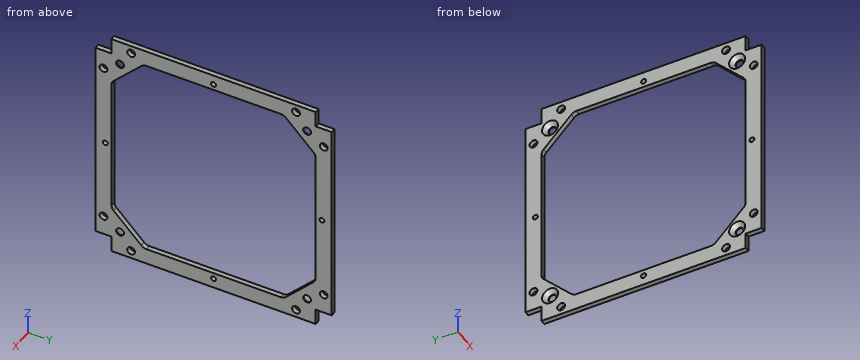
```python
from build123d import *

# Parameters (mm, degrees)
BOSS_EXTRUDE2_DEPTH                          = 2
F_3_2_3_2_DIAMETER_HOLE3_D                   = 3.2
CSK_FOR_M3_FLAT_COUNTERSUNK_HEAD_SCR_2_COUNT = 2
CSK_FOR_M3_FLAT_COUNTERSUNK_HEAD_SCR_2_PITCH = 76
CSK_FOR_M3_FLAT_COUNTERSUNK_HEAD_SCR_3_COUNT = 2
CSK_FOR_M3_FLAT_COUNTERSUNK_HEAD_SCR_3_PITCH = 107.48023074
CSK_FOR_M3_FLAT_COUNTERSUNK_HEAD_SCR_4_COUNT = 2
CSK_FOR_M3_FLAT_COUNTERSUNK_HEAD_SCR_4_PITCH = 76
M2_5X0_45_TAPPED_HOLE1_D                     = 2.05
FILLET1_R                                    = 3


with BuildPart() as part:
    # Sketch2 → Boss-Extrude2 (new body)
    with BuildSketch(Plane.ZY.offset(51.493641502)):
        Polygon((0.93465612, 3.45185693), (7.43465612, 3.45185693), (7.43465612, 86.45185693), (0.93465612, 86.45185693), (0.93465612, 92.95185693), (-82.06534388, 92.95185693), (-82.06534388, 86.45185693), (-88.56534388, 86.45185693), (-88.56534388, 3.45185693), (-82.06534388, 3.45185693), (-82.06534388, -3.04814307), (0.93465612, -3.04814307), align=None)
        Polygon((-82.06534388, 73.45185693), (-82.06534388, 16.45185693), (-69.06534388, 3.45185693), (-12.06534388, 3.45185693), (0.93465612, 16.45185693), (0.93465612, 73.45185693), (-12.06534388, 86.45185693), (-69.06534388, 86.45185693), align=None, mode=Mode.SUBTRACT)
    extrude(amount=BOSS_EXTRUDE2_DEPTH)

    # Ø3.2 (3.2) Diameter Hole3 (through all)
    with Locations(Plane.ZY.offset(53.493641502)):
        with Locations((-74.06534388, 0.20185693), (-85.31534388, 11.45185693), (-85.31534388, 78.45185693), (-74.06534388, 89.70185693), (-7.06534388, 89.70185693), (4.18465612, 78.45185693), (4.18465612, 11.45185693), (-7.06534388, 0.20185693)):
            Hole(F_3_2_3_2_DIAMETER_HOLE3_D / 2)

    # Sketch24 → CSK for M3 Flat Countersunk Head Screw5 (revolve, cut)
    with BuildSketch(Plane(origin=(-53.493641502, 6.95185693, -78.56534388), x_dir=(0, 0, 1), z_dir=(0, 1, 0))):
        Polygon((0, 0), (0, 2), (1.6, 2), (1.6, 1.65), (3.25, 0), align=None)
    csk_for_m3_flat_countersunk_head_screw5 = revolve(axis=Axis((-59.843641502, 6.95185693, -78.56534388), (1, 0, 0)), mode=Mode.SUBTRACT)

    # CSK for M3 Flat Countersunk Head Scr 2: CSK for M3 Flat Countersunk Head Screw5 ×2
    with Locations(*[(0, i * CSK_FOR_M3_FLAT_COUNTERSUNK_HEAD_SCR_2_PITCH, 0) for i in range(1, CSK_FOR_M3_FLAT_COUNTERSUNK_HEAD_SCR_2_COUNT)]):
        add(csk_for_m3_flat_countersunk_head_screw5, mode=Mode.SUBTRACT)

    # CSK for M3 Flat Countersunk Head Scr 3: CSK for M3 Flat Countersunk Head Screw5 ×2
    with Locations(*[Vector(0, 0.7071067811865478, 0.7071067811865472) * (i * CSK_FOR_M3_FLAT_COUNTERSUNK_HEAD_SCR_3_PITCH) for i in range(1, CSK_FOR_M3_FLAT_COUNTERSUNK_HEAD_SCR_3_COUNT)]):
        add(csk_for_m3_flat_countersunk_head_screw5, mode=Mode.SUBTRACT)

    # CSK for M3 Flat Countersunk Head Scr 4: CSK for M3 Flat Countersunk Head Screw5 ×2
    with Locations(*[(0, 0, i * CSK_FOR_M3_FLAT_COUNTERSUNK_HEAD_SCR_4_PITCH) for i in range(1, CSK_FOR_M3_FLAT_COUNTERSUNK_HEAD_SCR_4_COUNT)]):
        add(csk_for_m3_flat_countersunk_head_screw5, mode=Mode.SUBTRACT)

    # M2.5x0.45 Tapped Hole1 (through all)
    with Locations(Plane(origin=(-53.493641502, 88.95185693, -40.56534388), x_dir=(0, 0, -1), z_dir=(-1, 0, 0))):
        with Locations((0, 0), (44, 44), (0, 88), (-44, 44)):
            Hole(M2_5X0_45_TAPPED_HOLE1_D / 2)

    # Fillet1
    fillet1_edges = [part.edges().sort_by_distance(p)[0] for p in [
        (-52.493641502, 86.45185693, -69.06534388),
        (-52.493641502, 73.45185693, -82.06534388),
        (-52.493641502, 16.45185693, -82.06534388),
        (-52.493641502, 3.45185693, -69.06534388),
        (-52.493641502, 3.45185693, -12.06534388),
        (-52.493641502, 16.45185693, 0.93465612),
        (-52.493641502, 73.45185693, 0.93465612),
        (-52.493641502, 86.45185693, -12.06534388),
    ]]
    fillet(fillet1_edges, radius=FILLET1_R)


solid = part.part
```
CAD build for the part. Positions are in the model's coordinates, mm. Coordinates: 2 decimals unless noted, no trailing zeros. Write each loop counter-clockwise with the first axis right and the second up, starting at its lowest first coordinate (ties: lowest second). Pieces come first, ordered by that corner, then holes. Notation, with made-up numbers: (20.5, -14) -> (63.5, -14) arc R29 ccw to (63.5, 7) -> close; hole circle Ø5 at (40, -34.5). An arc over 180 degrees is marked (long way). Use CSV: the item, a comma, the result in double quotes. Start each with the question number.
Item 1: Band-saw the part on A-A, the plane y = 35.5. Write the cut outline in (x, z).
Item 2: Drop flat-ended pins along their axis: P1, Ø4, axis at y = 0.2, z = -74.07, coming from the +X side; P2, Ø0.6, axis at x = -52, z = 2.5, coming from the -Y side. Give the stop position or say it passes through.
Item 3: Band-saw the part on B-B, the plane z = -55. Write the cut outline in (x, y), plus the area to 3 significant figures.
Item 4: Band-saw the part on C-C, the plane x = -53.1. Give the number of separate pieces and of enclosed holes in the cut face, plus the area to 3 significant figures.
Item 5: Wall check: probe 1 along Y at (x, z) = (-51.8, -43); probe 2 along Z at (x, y) = (-52.45, 27); probe 3 along Y at (x, z) = (-52.7, -79.5). Give the ranges that are in metal, low to high.
Response values:
1,outline,"(-53.49, -88.57) -> (-51.49, -88.57) -> (-51.49, -82.07) -> (-53.49, -82.07) -> close; (-53.49, 0.93) -> (-51.49, 0.93) -> (-51.49, 7.43) -> (-53.49, 7.43) -> close"
2,P1,"stops at x = -51.49"
2,P2,"stops at y = 3.45"
3,outline,"(-53.49, -3.05) -> (-51.49, -3.05) -> (-51.49, 3.45) -> (-53.49, 3.45) -> close; (-53.49, 86.45) -> (-51.49, 86.45) -> (-51.49, 92.95) -> (-53.49, 92.95) -> close"
3,area,"26.0 mm2"
4,separate pieces,"1"
4,enclosed holes,"17"
4,area,"2,320 mm2"
5,probe 1,"y = -3.05 to 3.45, 86.45 to 92.95"
5,probe 2,"z = -88.57 to -82.07, 0.93 to 7.43"
5,probe 3,"y = -3.05 to 4.68, 9.22 to 13.89, 76.02 to 80.68, 85.22 to 92.95"
